```python
from build123d import *

# Parameters (mm, degrees)
CYLINDER001_R     = 4
CYLINDER001_DEPTH = 5
CYLINDER003_R     = 5.1
CYLINDER003_DEPTH = 5
FILLET_R          = 0.1


with BuildPart() as interior:
    # Cylinder001 → Cylinder001 (new body)
    with BuildSketch(Plane.XY):
        Circle(CYLINDER001_R)
    extrude(amount=CYLINDER001_DEPTH)


with BuildPart() as fillet_body:
    # Cylinder003 → Cylinder003 (new body)
    with BuildSketch(Plane.XY):
        Circle(CYLINDER003_R)
    extrude(amount=CYLINDER003_DEPTH)

    # Cut001: cut Interior
    add(interior.part, mode=Mode.SUBTRACT)

    # Fillet
    fillet_edges = [fillet_body.edges().sort_by_distance(p)[0] for p in [
        (-4, 0, 0),
        (-4, 0, 5),
    ]]
    fillet(fillet_edges, radius=FILLET_R)


solid = fillet_body.part
```
Input: part model. Units: mm. Frame: model coordinates. Give positions to 0.01 mm unless a question says otherwise; leave off trailing zeros. Order: outer loops, then holes, each group sorted by start corner. A loop starts at its lowest first (then second) coordinate and runs counter-clockwise, first axis right, second up. Notation, with made-up numbers: (-31.75, 19.25) -> (-2.75, 19.25) arc R37 cw to (-2.75, 56.25) -> close; hole circle Ø4 at (-6, 14.25). An arc over 180 degrees is marked (long way). Write each question's results on one line, items separated by ' | '. Start each with the question number.
Item 1: Mould query, pull axis X, two halves, no side actions, for faces 1 (the cylindrical face through (2.4, -4.5, 2.5)), 2 (the cylindrical face through (-0.867, -3.905, 2.466)). Classes: pulls with the +X half, pulls with the -X half, needs draft (parallel to the pull), parting line crosses it, or undercut.
Item 2: Cut plane A-A on x = 0. Return the cut outline in (y, z).
Item 3: Cut plane C-C on z = 3.85. Return the cut outline in (x, y).
Item 4: Line query: line 1 (Y direction, x = 0, z = 1.9); line 2 (X direction, y = -0.75, z = 3.2); line 3 (Y direction, x = -2.25, z = 2.5). Output: solid intervals per line, ascending.
Item 5: Contact query for a flat-ended pin moving along its axis: P1, Ø3, axis at x = 4, y = -2, coming from the -Z side. Output: stop coordinate, or through.
Established:
1) face 1: parting line crosses it | face 2: undercut
2) outline: (-5.1, 0) -> (-4.1, 0) arc R0.1 ccw to (-4, 0.1) -> (-4, 4.9) arc R0.1 ccw to (-4.1, 5) -> (-5.1, 5) -> close; (4, 0.1) arc R0.1 ccw to (4.1, 0) -> (5.1, 0) -> (5.1, 5) -> (4.1, 5) arc R0.1 ccw to (4, 4.9) -> close
3) outline: circle Ø10.2 at (0, 0); hole circle Ø8 at (0, 0)
4) line 1: -5.1 to -4, 4 to 5.1 | line 2: -5.04 to -3.93, 3.93 to 5.04 | line 3: -4.58 to -3.31, 3.31 to 4.58
5) P1: z = 0
